```python
from build123d import *

# Parameters (mm, degrees)
EXTRUDE_1_DEPTH     = 35
CUT_EXTRUDE_1_DEPTH = 22.5
SKETCH_5_R          = 1.3
CUT_EXTRUDE_3_DEPTH = 40.724048132
SKETCH_6_W          = 4.5
SKETCH_6_H          = 1.8
EXTRUDE_2_DEPTH     = 35


with BuildPart() as part:
    # 草圖2 → 填料-伸長1 (new body)
    with BuildSketch(Plane.XY):
        with BuildLine():
            Line((-8.5, -8), (8.5, -8))
            Line((8.5, -8), (8.5, 8))
            ThreePointArc((8.5, 8), (0, 6.967375879), (-8.5, 8))
            Line((-8.5, 8), (-8.5, -8))
        make_face()
    extrude(amount=-EXTRUDE_1_DEPTH)

    # 草圖3 → 除料-伸長1 (cut)
    with BuildSketch(Plane.XY):
        with BuildLine():
            Line((-3.4, -8), (3.4, -8))
            Line((3.4, -8), (3.4, 7.130567874))
            ThreePointArc((3.4, 7.130567874), (0, 6.967375879), (-3.4, 7.130567874))
            Line((-3.4, 7.130567874), (-3.4, -8))
        make_face()
    extrude(amount=-CUT_EXTRUDE_1_DEPTH, mode=Mode.SUBTRACT)

    # 草圖5 → 除料-伸長3 (cut, through all)
    with BuildSketch(Plane.ZY.offset(8.5)):
        with Locations((-5.2, -4.1)):
            Circle(SKETCH_5_R)
        with Locations((-14.7, -4.1)):
            Circle(SKETCH_5_R)
    extrude(amount=-CUT_EXTRUDE_3_DEPTH, mode=Mode.SUBTRACT)

    # 草圖6 → 填料-伸長2 (add)
    with BuildSketch(Plane.XY):
        with Locations((10.75, 4.6)):
            Rectangle(SKETCH_6_W, SKETCH_6_H)
    extrude_2 = extrude(amount=-EXTRUDE_2_DEPTH)

    # 鏡射1: 填料-伸長2 across plane
    add(extrude_2.mirror(Plane(origin=(0, 0, 0), x_dir=(0, 0, 1), z_dir=(1, 0, 0))))


solid = part.part
```
The listing builds one solid part. Answer for the finished solid, in the listing's coordinates (mm). A direction names the side the tool comes from. Round coordinates to 2 decimals unless told otherwise and drop trailing zeros. Loops run counter-clockwise (first coordinate to the right, second up) from the corner with the lowest first, then second, coordinate; pieces in that order, holes last.
1) Given P1, Ø4, axis at y = -4.1, z = -5.2, coming from the +X side; P2, Ø2, axis at x = -11.5, z = -18, coming from the -Y side; P3, Ø3.5, axis at x = 0, y = -2.5, coming from the +Z side, each flat-ended and moving along its own axis, determine where each tip first touches the part or whether it passes through.
Outcome:
P1: stops at x = 8.5
P2: stops at y = 3.7
P3: stops at z = -22.5
2) Consider line 1 (X direction, y = 1.25, z = -3.5); line 2 (Z direction, x = -4.75, y = -3.5); line 3 (Z direction, x = -4.5, y = -3). Determine where each line is inside the solid, lowest interval first.
Outcome:
line 1: x = -8.5 to -3.4, 3.4 to 8.5
line 2: z = -35 to -15.85, -13.55 to -6.35, -4.05 to 0
line 3: z = -35 to -15.39, -14.01 to -5.89, -4.51 to 0
3) A cutting plane is placed at D-D on x = 5.5. Determine the outline of the cut face in (y, z).
Outcome:
outline: (-8, -35) - (7.4, -35) - (7.4, 0) - (-8, 0) - close; hole circle Ø2.6 at (-4.1, -14.7); hole circle Ø2.6 at (-4.1, -5.2)
4) A cutting plane is placed at A-A on z = -14.7. Determine the outline of the cut face in (x, y), plus the area to 3 significant figures.
Outcome:
outline: (-13, 3.7) - (-8.5, 3.7) - (-8.5, -2.8) - (-3.4, -2.8) - (-3.4, 7.13) arc R35.5 cw to (-8.5, 8) - (-8.5, 5.5) - (-13, 5.5) - close; (-8.5, -8) - (-3.4, -8) - (-3.4, -5.4) - (-8.5, -5.4) - close; (3.4, -8) - (8.5, -8) - (8.5, -5.4) - (3.4, -5.4) - close; (3.4, -2.8) - (8.5, -2.8) - (8.5, 3.7) - (13, 3.7) - (13, 5.5) - (8.5, 5.5) - (8.5, 8) arc R35.5 cw to (3.4, 7.13) - close
area: 148 mm2
5) A cutting plane is placed at C-C on z = -28. Determine the outline of the cut face in (x, y), plus the area to 3 significant figures.
Outcome:
outline: (-13, 3.7) - (-8.5, 3.7) - (-8.5, -8) - (8.5, -8) - (8.5, 3.7) - (13, 3.7) - (13, 5.5) - (8.5, 5.5) - (8.5, 8) arc R35.5 cw to (-8.5, 8) - (-8.5, 5.5) - (-13, 5.5) - close
area: 276 mm2
6) For a pull along X with two mould halves and no side action, classify faces 1 (the face through (-13, 5, -17)), 2 (the face through (5.91, -2.81, -5.37)), 3 (the face through (3.927, 7.185, -17.255)), 4 (the face through (13, 5, -17)) as released by +X, released by -X, zero draft, split by the parting line, or undercut.
Outcome:
face 1: released by -X
face 2: zero draft
face 3: undercut
face 4: released by +X
7) For faces 5 (the face through (11, 5.5, -17)), 6 (the face through (0, 0, -22.5)), 7 (the face through (-8.5, 7, -17)), 8 (the face through (11, 3.7, -17)), determine the directions among +Z, -Z, +X, -X, +Y, -Y from which every point of the face is accessible in a straight line to the end or side of a thin tool.
Outcome:
face 5: +Z, -Z, +X, +Y
face 6: +Z, +Y, -Y
face 7: +Z, -Z, -X, +Y
face 8: +Z, -Z, +X, -Y
8) A cutting plane is placed at B-B on y = -4.1. Determine the outline of the cut face in (x, z), plus the area to 3 significant figures.
Outcome:
outline: (-8.5, -35) - (8.5, -35) - (8.5, -16) - (3.4, -16) - (3.4, -22.5) - (-3.4, -22.5) - (-3.4, -16) - (-8.5, -16) - close; (-8.5, -13.4) - (-3.4, -13.4) - (-3.4, -6.5) - (-8.5, -6.5) - close; (-8.5, -3.9) - (-3.4, -3.9) - (-3.4, 0) - (-8.5, 0) - close; (3.4, -13.4) - (8.5, -13.4) - (8.5, -6.5) - (3.4, -6.5) - close; (3.4, -3.9) - (8.5, -3.9) - (8.5, 0) - (3.4, 0) - close
area: 389 mm2
